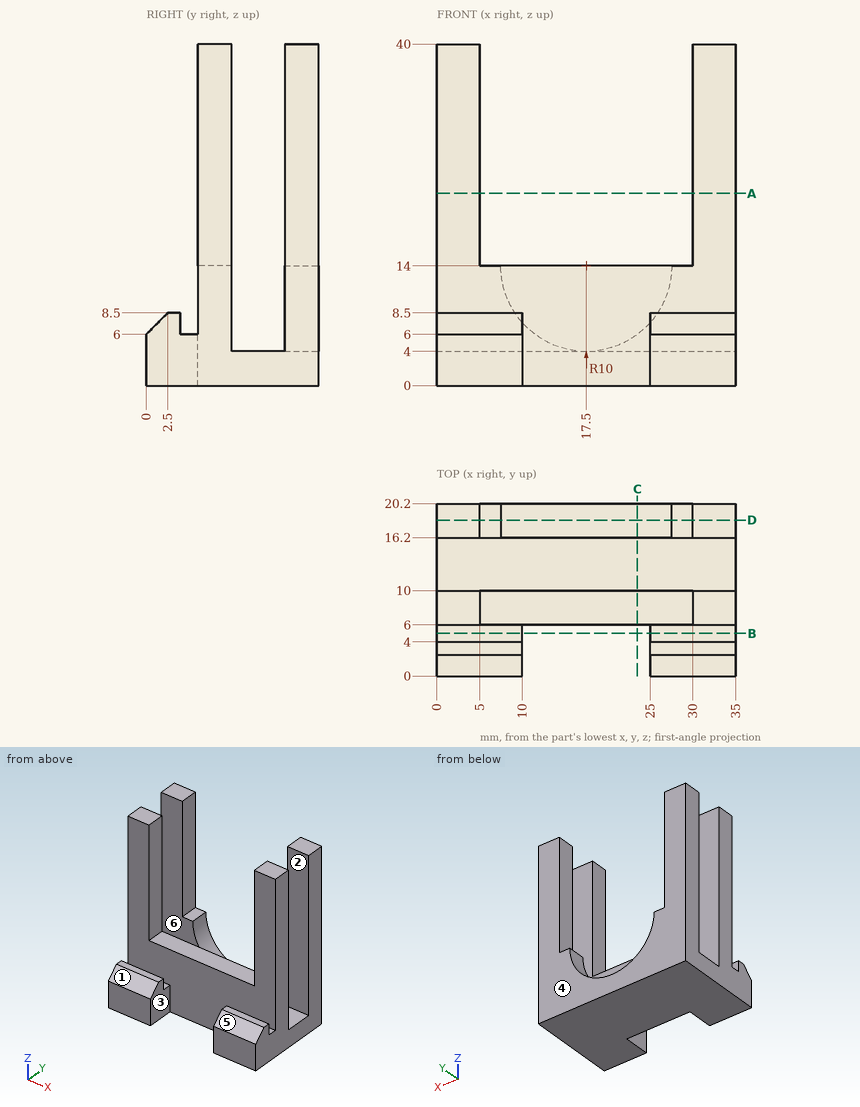
Source: three-view drawing plus pictorial views. Frame: mm from the lowest corner of the part. A direction names the side the tool comes from. Give positions to 0.01 mm unless a question says otherwise; leave off trailing zeros. Write each loop counter-clockwise with the first axis right and the second up, starting at its lowest first coordinate (ties: lowest second). Pieces come first, ordered by that corner, then holes. Notation, with made-up numbers: (-22.5, 46.25) -> (14.5, 46.25) arc R22 ccw to (14.5, 82.25) -> close; hole circle Ø6 at (62, -18). An arc over 180 degrees is marked (long way). Answer in a Markdown table with one row per item.
(1) Section query C-C on x = 23.5. Return loops of the section in (y, z).
Answers below:
| item | result |
|---|---|
| outline | (6, 0) -> (20.2, 0) -> (20.2, 6) -> (16.2, 6) -> (16.2, 4) -> (10, 4) -> (10, 14) -> (6, 14) -> close |
(2) Section query B-B on y = 5. Return loops of the section in (x, z).
Answers below:
| item | result |
|---|---|
| outline | (0, 0) -> (10, 0) -> (10, 6) -> (0, 6) -> close; (25, 0) -> (35, 0) -> (35, 6) -> (25, 6) -> close |
(3) Draft query along Y for the marked faces 4, 5 and 6. Return one class per face: +Y half, -Y half, draft (parallel to the pull), parting line (faces both ways), or undercut.
Answers below:
| item | result |
|---|---|
| face 4 | +Y half |
| face 5 | -Y half |
| face 6 | undercut |
(4) Section query D-D on y = 18.25. Return loops of the section in (x, z).
Answers below:
| item | result |
|---|---|
| outline | (0, 0) -> (35, 0) -> (35, 40) -> (30, 40) -> (30, 14) -> (27.5, 14) arc R10 cw to (7.5, 14) -> (5, 14) -> (5, 40) -> (0, 40) -> close |
(5) Ray query, line 1 along X through (y, z) = (8, 37.5); line 2 along Y through (x, z) = (29, 4.5); line 3 along Y through (x, z) = (10.5, 6). Return the intervals inside material, ascending. Write a range as [from, to].
Answers below:
| item | result |
|---|---|
| line 1 | [0, 5], [30, 35] |
| line 2 | [0, 10], [16.2, 20.2] |
| line 3 | [6, 10], [16.2, 20.2] |
(6) Section query A-A on z = 22.5. Return loops of the section in (x, y).
Answers below:
| item | result |
|---|---|
| outline | (0, 6) -> (5, 6) -> (5, 10) -> (0, 10) -> close; (0, 16.2) -> (5, 16.2) -> (5, 20.2) -> (0, 20.2) -> close; (30, 6) -> (35, 6) -> (35, 10) -> (30, 10) -> close; (30, 16.2) -> (35, 16.2) -> (35, 20.2) -> (30, 20.2) -> close |
(7) Pin query (flat end, axial travel): pin 1 (4 mm diameter, centred on x = 18.5, y = 14, fed in from +Z); pin 2 (5 mm diameter, centred on x = 28.5, z = 19.5, fed in from -Y); pin 3 (0.8 mm diameter, centred on x = 28.5, y = 3.5, fed in from +Z). Return the tip coordinate at first contact, or that it passes through.
Answers below:
| item | result |
|---|---|
| pin 1 | z = 4 |
| pin 2 | y = 6 |
| pin 3 | z = 8.5 |
(8) Set-up query: the marked faces 1, 2 and 3. Return all of +Z, -Z, +X, -X, +Y, -Y with unobstructed straight access to the full face (end or side cutting, diameter ignored); none if empty.
Answers below:
| item | result |
|---|---|
| face 1 | +Z, +X, -X, -Y |
| face 2 | +Z, +X, -X |
| face 3 | +Z, -Z, -Y |
